Input: part model. Units: mm. Frame: model coordinates. A direction names the side the tool comes from. Give positions to 0.01 mm unless a question says otherwise; leave off trailing zeros. Loops run counter-clockwise (first coordinate to the right, second up) from the corner with the lowest first, then second, coordinate; pieces in that order, holes last.
from build123d import *

# Parameters (mm, degrees)
BOSS_EXTRUDE1_DEPTH = 15
SHELL1_T            = -4
CUT_EXTRUDE1_DEPTH  = 15
SKETCH3_R           = 1
CUT_EXTRUDE2_DEPTH  = 6
FILLET1_R           = 0.5
SKETCH4_R           = 2
CUT_EXTRUDE3_DEPTH  = 116.95257659
CHAMFER1_SIZE       = 1
CUT_EXTRUDE7_DEPTH  = 88.389930872
SKETCH9_R           = 1.6
BOSS_EXTRUDE3_DEPTH = 4
SKETCH10_R          = 4.5
CUT_EXTRUDE8_DEPTH  = 10
FILLET2_R           = 1


with BuildPart() as part:
    # Sketch1 → Boss-Extrude1 (new body)
    with BuildSketch(Plane(origin=(0, 0, 0), x_dir=(1, 0, 0), z_dir=(0, 1, 0))):
        with BuildLine():
            Line((-30, 44), (30, 44))
            ThreePointArc((30, 44), (74, 0), (30, -44))
            Line((30, -44), (-30, -44))
            ThreePointArc((-30, -44), (-74, 0), (-30, 44))
        make_face()
    extrude(amount=BOSS_EXTRUDE1_DEPTH)

    # Shell1
    shell1_openings = [part.faces().sort_by_distance(p)[0] for p in [
        (0, 15, 0),
    ]]
    offset(amount=SHELL1_T, openings=shell1_openings, kind=Kind.INTERSECTION)

    # Sketch2 → Cut-Extrude1 (cut)
    with BuildSketch(Plane(origin=(0, 4, 0), x_dir=(1, 0, 0), z_dir=(0, 1, 0))):
        with BuildLine():
            Line((-30, -24), (30, -24))
            ThreePointArc((30, -24), (35, -29), (30, -34))
            Line((30, -34), (-30, -34))
            ThreePointArc((-30, -34), (-35, -29), (-30, -24))
        make_face()
    extrude(amount=-CUT_EXTRUDE1_DEPTH, mode=Mode.SUBTRACT)

    # Sketch3 → Cut-Extrude2 (cut)
    with BuildSketch(Plane(origin=(0, 15, 0), x_dir=(1, 0, 0), z_dir=(0, 1, 0))):
        with Locations(Location((-30, -42, 0), (0, 0, 270))):
            Circle(SKETCH3_R)
        with Locations(Location((0, -42, 0), (0, 0, 270))):
            Circle(SKETCH3_R)
        with Locations(Location((30, -42, 0), (0, 0, 270))):
            Circle(SKETCH3_R)
        with Locations(Location((-30, 42, 0), (0, 0, 270))):
            Circle(SKETCH3_R)
        with Locations(Location((0, 42, 0), (0, 0, 270))):
            Circle(SKETCH3_R)
        with Locations(Location((30, 42, 0), (0, 0, 270))):
            Circle(SKETCH3_R)
        with Locations(Location((66.105117767, 22, 0), (0, 0, 270))):
            Circle(SKETCH3_R)
        with Locations(Location((72, 0, 0), (0, 0, 270))):
            Circle(SKETCH3_R)
        with Locations(Location((-66.105117767, 22, 0), (0, 0, 270))):
            Circle(SKETCH3_R)
        with Locations(Location((-72, 0, 0), (0, 0, 270))):
            Circle(SKETCH3_R)
        with Locations(Location((-66.105117767, -22, 0), (0, 0, 270))):
            Circle(SKETCH3_R)
        with Locations(Location((66.105117767, -22, 0), (0, 0, 270))):
            Circle(SKETCH3_R)
    extrude(amount=-CUT_EXTRUDE2_DEPTH, mode=Mode.SUBTRACT)

    # Fillet1
    fillet1_edges = [part.edges().sort_by_distance(p)[0] for p in [
        (-74, 15, 0),
        (70, 15, 0),
        (0, 15, -40),
        (-70, 15, 0),
        (0, 15, 44),
        (0, 15, 40),
        (74, 15, 0),
        (0, 15, -44),
    ]]
    fillet(fillet1_edges, radius=FILLET1_R)

    # Sketch4 → Cut-Extrude3 (cut, through all)
    with BuildSketch(Plane.XY.offset(44)):
        with Locations((-20, 7.25)):
            Circle(SKETCH4_R)
        with Locations(Location((20, 7.25, 0), (0, 0, 180))):
            Circle(SKETCH4_R)
    extrude(amount=-CUT_EXTRUDE3_DEPTH, mode=Mode.SUBTRACT)

    # Chamfer1
    chamfer1_edges = [part.edges().sort_by_distance(p)[0] for p in [
        (-35, 4, 29),
        (0, 4, 34),
        (35, 4, 29),
        (0, 4, 24),
    ]]
    chamfer(chamfer1_edges, length=CHAMFER1_SIZE)

    # Sketch6 → Cut-Extrude7 (cut, through all)
    with BuildSketch(Plane(origin=(0, 0, 0), x_dir=(1, 0, 0), z_dir=(0, 1, 0))):
        with BuildLine():
            Line((83, 15), (67.080992435, 15))
            ThreePointArc((67.080992435, 15), (70, 0), (67.080992435, -15))
            Line((67.080992435, -15), (83, -15))
            Line((83, -15), (83, 15))
        make_face()
    extrude(amount=CUT_EXTRUDE7_DEPTH, mode=Mode.SUBTRACT)

    # Sketch9 → Boss-Extrude3 (add)
    with BuildSketch(Plane(origin=(0, 4, 0), x_dir=(1, 0, 0), z_dir=(0, 1, 0))):
        with Locations(Location((33.03, 16.83, 0), (0, 0, 270))):
            Circle(SKETCH9_R)
        with Locations(Location((33.03, -11.34, 0), (0, 0, 270))):
            Circle(SKETCH9_R)
        with Locations(Location((-17.78, 32.16, 0), (0, 0, 270))):
            Circle(SKETCH9_R)
        with Locations(Location((-19.03, -16.16, 0), (0, 0, 270))):
            Circle(SKETCH9_R)
    extrude(amount=BOSS_EXTRUDE3_DEPTH)

    # Sketch10 → Cut-Extrude8 (cut)
    with BuildSketch(Plane(origin=(0, 4, 0), x_dir=(1, 0, 0), z_dir=(0, 1, 0))):
        with Locations(Location((50, 0, 0), (0, 0, 270))):
            Circle(SKETCH10_R)
        with Locations(Location((-50, 0, 0), (0, 0, 270))):
            Circle(SKETCH10_R)
    extrude(amount=-CUT_EXTRUDE8_DEPTH, mode=Mode.SUBTRACT)

    # Fillet2
    fillet2_edges = [part.edges().sort_by_distance(p)[0] for p in [
        (50, 4, -4.5),
        (-50, 4, -4.5),
    ]]
    fillet(fillet2_edges, radius=FILLET2_R)


solid = part.part
(1) Pin query (flat end, axial travel): pin 1 Ø4 at (x, y) = (35.5, 8.5) entering from -Z; pin 2 Ø1.5 at (x, z) = (8.5, 33) entering from +Y; pin 3 Ø1.6 at (x, z) = (30, 42) entering from +Y; pin 4 Ø5 at (x, y) = (41.5, 11.5) entering from -Z. Return the tip coordinate at first contact, or that it passes through.
Values follow:
pin 1: stops at z = -43.86
pin 2: passes through
pin 3: stops at y = 9
pin 4: stops at z = -43.07
(2) Mould query, pull axis Y, two halves, no side actions, for faces 1 (the cylindrical face through (21.587, 8.467, 42.028)), 2 (the cylindrical face through (-21.474, 8.602, -41.972)), 3 (the conical face through (35.2, 3.2, 28.9)), 4 (the cylindrical face through (55.566, 7.148, 35.81)). Classes: +Y half, -Y half, draft (parallel to the pull), parting line (faces both ways), or undercut.
Values follow:
face 1: undercut
face 2: undercut
face 3: +Y half
face 4: draft
(3) Ray query, probe 1 along X at (y, z) = (1.95, 0); probe 2 along Y at (x, z) = (20, -41.3); probe 3 along Z at (x, y) = (-65.5, 12). Return the intervals inside material, ascending.
Values follow:
probe 1: x = -74 to -54.5, -45.5 to 45.5, 54.5 to 70
probe 2: y = 0 to 5.25, 9.25 to 15
probe 3: z = -26 to -22.8, -21.2 to -18.43, 18.43 to 21.2, 22.8 to 26
(4) Reachability of faces 5 (the flat face through (0, 7, -44)), 6 (the flat face through (-18, 8, -32)), 7 (the flat face through (69, 7, 15)), 8 (the flat face through (0, 2, 34)), 9 (the cylindrical face through (-73.99, 7.15, 0.97)) from +Z, -Z, +X, -X, +Y, -Y: full face, straight path, thin tool, end or side. Return the list, or none.
Values follow:
face 5: -Z, +X, -X, +Y, -Y
face 6: +Y
face 7: +X, +Y, -Y
face 8: +Y, -Y
face 9: -X, +Y, -Y
(5) Cut plane A-A (x = 8.5). Return the cut outline in (y, z), and give its area (3 significant figures).
Values follow:
outline: (0, -44) - (14.5, -44) arc R0.5 ccw to (15, -43.5) - (15, -40.5) arc R0.5 ccw to (14.5, -40) - (4, -40) - (4, 23) - (3, 24) - (0, 24) - close; (0, 34) - (3, 34) - (4, 35) - (4, 40) - (14.5, 40) arc R0.5 ccw to (15, 40.5) - (15, 43.5) arc R0.5 ccw to (14.5, 44) - (0, 44) - close
area: 399 mm2
